```python
from build123d import *

# Parameters (mm, degrees)
F3_R = 3
F4_R = 1


# Not quite as in the source:
# - a fillet or chamfer that OpenCascade refuses, or shapes differently, is made with other operations: its cross-section is extruded or revolved along the edge and cut away or added


with BuildPart() as f1:
    # F0 (on Top) → F1 (revolve)
    with BuildSketch(Plane.XY):
        Polygon((-30, 26.65), (0, 26.65), (0, 37.5), (-3, 37.5), (-3, 29.65), (-27, 29.65), (-27, 37.5), (-30, 37.5), align=None)
    revolve(axis=Axis((5.0713585872, 0, 0), (1, 0, 0)))

    # F2: fillet of radius 8 on 1 edges, made by hand

    # F2_s1 → F2_t2 (revolve)
    with BuildSketch(Plane.XY):
        with BuildLine():
            ThreePointArc((-19.0014063736, 29.65), (-24.6049766641, 31.9403590306), (-27, 37.5))
            Line((-27, 37.5), (-27, 29.65))
            Line((-27, 29.65), (-19.0014063736, 29.65))
        make_face()
    revolve(axis=Axis((-27, 0, 0), (1, 0, 0)))

    # F3
    f3_edges = [f1.edges().sort_by_distance(p)[0] for p in [
        (0, -26.65, 0),
        (-30, -26.65, 0),
    ]]
    fillet(f3_edges, radius=F3_R)

    # F4
    f4_edges = [f1.edges().sort_by_distance(p)[0] for p in [
        (-3, -29.65, 0),
    ]]
    fillet(f4_edges, radius=F4_R)


solid = f1.part
```
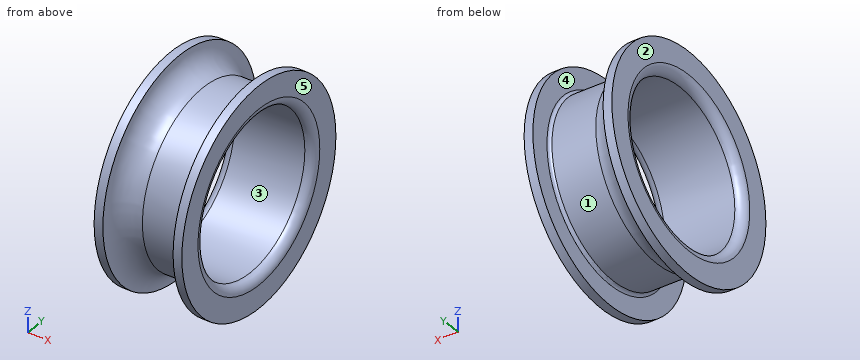
Check sheet for the modelled part. Datum: model origin and axes. Units: mm. Face numbers are marked on the shaded views. A direction names the side the tool comes from. Coordinates: 2 decimals unless noted, no trailing zeros. Order: outer loops, then holes, each group sorted by start corner. A loop starts at its lowest first (then second) coordinate and runs counter-clockwise, first axis right, second up. Notation, with made-up numbers: (-23.75, 50.25) -> (35.25, 50.25) arc R33 cw to (35.25, 79.25) -> close; hole circle Ø1 at (58, 0.5). An arc over 180 degrees is marked (long way). Write item = value, one per line. Start each with the question number.
1) Access from +Z, -Z, +X, -X, +Y, -Y to the whole of each face (thin tool, end or side, straight path). Record for the marked faces 1 and 2.
2) Cross-section at C-C (x = -13). Enter the section's corners in (y, z), then the cut area to 3 significant figures.
3) Material ranges on L1, parallel to Z at x = -10.5, y = 0; L2, parallel to Y at x = -24.5, z = -5; L3, parallel to Z at x = -19.5, y = -15.5, recorded low to high.
4) Cross-section at A-A (y = 0). Enter the section's corners in (x, z), then the cut area to 3 significant figures.
5) Go/stop test with flat-tipped pins: P1, Ø2, axis at x = -14, z = -7.5, coming from the +Y side; P2, Ø3, axis at x = -12, z = 2.5, coming from the +Y side; P3, Ø8, axis at x = -17.5, z = -15, coming from the -Y side. Record where each tip stops, or that it passes through.
6) Mould release check, pull along X, two halves, no side actions. Record for the marked faces 3, 4 and 5: +X half, -X half, draft (parallel to the pull), parting line (faces both ways), or undercut.
7) Cross-section at D-D (x = -22). Enter the section's corners in (y, z).
Ans:
q1.face_1 = none
q1.face_2 = +Z, -Z, -X, +Y, -Y
q2.outline = circle Ø59.3 at (0, 0); hole circle Ø53.3 at (0, 0)
q2.area = 531 mm²
q3.L1 = -29.65 to -26.65, 26.65 to 29.65
q3.L2 = -31.44 to -26.18, 26.18 to 31.44
q3.L3 = -25.29 to -21.68, 21.68 to 25.29
q4.outline = (-30, -37.5) -> (-27, -37.5) arc R8 cw to (-19, -29.65) -> (-4, -29.65) arc R1 cw to (-3, -30.65) -> (-3, -37.5) -> (0, -37.5) -> (0, -29.65) arc R3 ccw to (-3, -26.65) -> (-27, -26.65) arc R3 ccw to (-30, -29.65) -> close; (-30, 29.65) arc R3 ccw to (-27, 26.65) -> (-3, 26.65) arc R3 ccw to (0, 29.65) -> (0, 37.5) -> (-3, 37.5) -> (-3, 30.65) arc R1 cw to (-4, 29.65) -> (-19, 29.65) arc R8 cw to (-27, 37.5) -> (-30, 37.5) -> close
q4.area = 294 mm²
q5.P1 = 28.93
q5.P2 = 29.63
q5.P3 = -27.53
q6.face_3 = draft
q6.face_4 = undercut
q6.face_5 = +X half
q7.outline = circle Ø60.47 at (0, 0); hole circle Ø53.3 at (0, 0)
